```python
from build123d import *
from build123d.topology import SkipClean

# Parameters (mm, degrees)
SKETCH3_R           = 7.5
BOSS_EXTRUDE1_DEPTH = 2


with BuildPart() as part:
    # Sketch3 → Boss-Extrude1 (new body)
    with BuildSketch(Plane(origin=(0, 0, 0), x_dir=(1, 0, 0), z_dir=(0, 1, 0))):
        with Locations(Location((0, 0, 0), (0, 0, 270))):
            Circle(SKETCH3_R)
    extrude(amount=-BOSS_EXTRUDE1_DEPTH)

    # Sketch4 → Revolve3 (revolve)
    with BuildSketch(Plane.XY):
        Polygon((0, -2), (0, -19), (-2.45, -19), (-2.45, -17), (-1.2, -17), (-1.2, -6), (-2.5, -6), (-2.5, -4.5), (-1.2, -4.5), (-1.2, -4), (-4, -2), align=None)
    revolve(axis=Axis((0, -2, 0), (0, -1, 0)))

    # Sketch5 → Revolve4 (revolve)
    with SkipClean():  # the faces are left unmerged after this step: merging them gives an invalid solid
        with BuildSketch(Plane(origin=(0, 0, 0), x_dir=(0, 0, -1), z_dir=(1, 0, 0)), mode=Mode.PRIVATE) as revolve4_sk:
            with BuildLine():
                ThreePointArc((-1.5, 3.4), (-0.764852927, 3.175735365), (0, 3.1))
                Line((0, 3.1), (0, 7))
                Line((0, 7), (0, 10.9))
                ThreePointArc((0, 10.9), (-3.824264635, 7.764852927), (-1.5, 3.4))
            make_face()
            with BuildLine():
                Line((0, 7), (0, 3.1))
                ThreePointArc((0, 3.1), (0.764852927, 3.175735365), (1.5, 3.4))
                ThreePointArc((1.5, 3.4), (3.244996148, 4.836669235), (3.9, 7))
                ThreePointArc((3.9, 7), (2.757716447, 9.757716447), (0, 10.9))
                Line((0, 10.9), (0, 7))
            make_face()
            with BuildLine():
                Line((-1.5, 0), (0, 0))
                Line((0, 0), (0, 3.1))
                ThreePointArc((0, 3.1), (-0.764852927, 3.175735365), (-1.5, 3.4))
                Line((-1.5, 3.4), (-1.5, 0))
            make_face()
        revolve(revolve4_sk.sketch.rotate(Axis((0, 10.9, 0), (0, -1, 0)), 180), axis=Axis((0, 10.9, 0), (0, -1, 0)))


solid = part.part
```
CAD build for the part. Positions are in the model's coordinates, mm. A direction names the side the tool comes from. Give positions to 0.01 mm unless a question says otherwise; leave off trailing zeros. Loops run counter-clockwise (first coordinate to the right, second up) from the corner with the lowest first, then second, coordinate; pieces in that order, holes last. Notation, with made-up numbers: (41.25, 7.5) - (78.25, 7.5) arc R4 ccw to (78.25, 12.5) - close; hole circle Ø5 at (60, 10.25). An arc over 180 degrees is marked (long way). Put each result on its own line as item: value.
Q1. Probe line 1 along Y through (x, z) = (5.5, -3.25); line 2 along Y through (x, z) = (-1.5, 1.5); line 3 along Y through (x, z) = (-0.5, -3.5). List the from-to ranges inside material, lowest first.
Filled in:
line 1: y = -2 to 0
line 2: y = -19 to -17, -6 to -4.5, -3.34 to 0, 3.73 to 10.27
line 3: y = -2.33 to 0, 5.35 to 8.65
Q2. Mould opens along Y. For faces 1 (the face through (0.298, -3.875, 1.342)), 2 (the face through (0.54, -5.24, 2.44)), 3 (the face through (0.45, 1.68, -1.43)), 4 (the face through (0, -19, 0)) say: pulls with the +Y half, pulls with the -Y half, needs draft (parallel to the pull), parting line crosses it, or undercut.
Filled in:
face 1: undercut
face 2: needs draft
face 3: undercut
face 4: pulls with the -Y half
Q3. Tool access for faces 5 (the face through (-1, -4.5, -1)), 6 (the face through (-3, -2, 3)), 7 (the face through (0.33, -0.986, -7.493)): list every direction of +Z, -Z, +X, -X, +Y, -Y with a clear straight run to the whole face (end or side of a thin tool).
Filled in:
face 5: none
face 6: -Y
face 7: +Y, -Y
Q4. Slice it at A-A (z = 0). Give the cut face in (x, y), plus the area to 3 significant figures.
Filled in:
outline: (-7.5, -2) - (-4, -2) - (-1.2, -4) - (-1.2, -4.5) - (-2.5, -4.5) - (-2.5, -6) - (-1.2, -6) - (-1.2, -17) - (-2.45, -17) - (-2.45, -19) - (2.45, -19) - (2.45, -17) - (1.2, -17) - (1.2, -6) - (2.5, -6) - (2.5, -4.5) - (1.2, -4.5) - (1.2, -4) - (4, -2) - (7.5, -2) - (7.5, 0) - (1.5, 0) - (1.5, 3.4) arc R3.9 ccw (long way) to (-1.5, 3.4) - (-1.5, 0) - (-7.5, 0) - close
area: 143 mm²
Q5. Slice it at B-B (x = 0). Give the cut face in (y, z), plus the area to 3 significant figures.
Filled in:
outline: (-19, -2.45) - (-17, -2.45) - (-17, -1.2) - (-6, -1.2) - (-6, -2.5) - (-4.5, -2.5) - (-4.5, -1.2) - (-4, -1.2) - (-2, -4) - (-2, -7.5) - (0, -7.5) - (0, -1.5) - (3.4, -1.5) arc R3.9 ccw (long way) to (3.4, 1.5) - (0, 1.5) - (0, 7.5) - (-2, 7.5) - (-2, 4) - (-4, 1.2) - (-4.5, 1.2) - (-4.5, 2.5) - (-6, 2.5) - (-6, 1.2) - (-17, 1.2) - (-17, 2.45) - (-19, 2.45) - close
area: 143 mm²
Q6. Flat gauge pins, fed straight in: pin 1 (2 mm diameter, centred on x = -6, y = -1, fed in from -Z); pin 2 (1.5 mm diameter, centred on x = -1, y = -4.5, fed in from -Z); pin 3 (6 mm diameter, centred on x = 1.5, z = -3, fed in from +Y); pin 4 (5 mm diameter, centred on y = -15.5, z = 5.5, fed in from +X). Where does each tip first touch, or does it go through?
Filled in:
pin 1: stops at z = -5.59
pin 2: stops at z = -2.49
pin 3: stops at y = 10.88
pin 4: passes through
Q7. Slice it at C-C (y = 2.5). Give the cut face in (x, z).
Filled in:
outline: circle Ø3 at (0, 0)
Q8. Slice it at D-D (y = -9.25). Give the cut face in (x, z).
Filled in:
outline: circle Ø2.4 at (0, 0)
